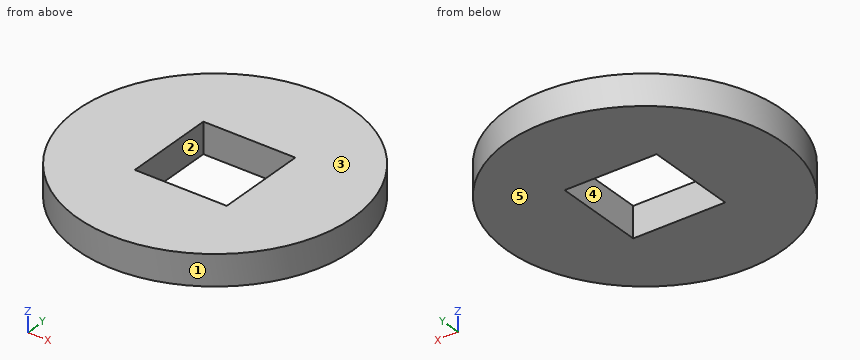
from build123d import *

# Parameters (mm, degrees)
SKETCH_1_R      = 4.5
SKETCH_1_W      = 3
SKETCH_1_H      = 3
EXTRUDE_1_DEPTH = 1


with BuildPart() as part:
    # 草图1 → 凸台-拉伸1 (new body)
    with BuildSketch(Plane.XY):
        Circle(SKETCH_1_R)
        Rectangle(SKETCH_1_W, SKETCH_1_H, mode=Mode.SUBTRACT)
    extrude(amount=EXTRUDE_1_DEPTH)


solid = part.part
Build history of the part. All positions in model axes, mm. Face numbers are marked on the shaded views. A direction names the side the tool comes from. Give positions to 0.01 mm unless a question says otherwise; leave off trailing zeros. Order: outer loops, then holes, each group sorted by start corner. A loop starts at its lowest first (then second) coordinate and runs counter-clockwise, first axis right, second up. Notation, with made-up numbers: M -18.5,20.25 L 7.5,20.25 A18 cw 7.5,42.25 Z; hole C -28,49.25 d1. An arc over 180 degrees is marked long. Put each result on its own line as item: value.
Item 1: Slice it at C-C, the plane z = 0.7. Write the cut outline in (x, y), plus the area to 3 significant figures.
From the geometry:
outline: C 0,0 d9; hole M -1.5,-1.5 L 1.5,-1.5 L 1.5,1.5 L -1.5,1.5 Z
area: 54.6 mm2
Item 2: Two-plate mould, pull along Y, no slides. Class the marked faces 1, 2 and 3: +Y half, -Y half, draft (parallel to the pull), parting line (faces both ways), or undercut.
From the geometry:
face 1: parting line
face 2: undercut
face 3: draft
Item 3: Flat gauge pin, fed straight in: pin 1 Ø5 at (x, y) = (-2.5, 2.5) entering from -Z. Where does the tip first touch, or does it go through?
From the geometry:
pin 1: stops at z = 0
Item 4: Probe line 1 (Y direction, x = -1, z = 0.6); line 2 (Y direction, x = 0, z = 0.8); line 3 (X direction, y = 0.25, z = 0.6). List the from-to ranges inside material, lowest first. Write a range as [from, to].
From the geometry:
line 1: y = [-4.39, -1.5], [1.5, 4.39]
line 2: y = [-4.5, -1.5], [1.5, 4.5]
line 3: x = [-4.49, -1.5], [1.5, 4.49]
Item 5: 3-axis set-ups, long thin cutter, end or side, ignore diameter. For the marked faces 4 and 5: which of +Z, -Z, +X, -X, +Y, -Y reach the whole face in a straight line?
From the geometry:
face 4: +Z, -Z
face 5: -Z, +X, -X, +Y, -Y
Item 6: Slice it at A-A, the plane y = 0. Write the cut outline in (x, z), plus the area to 3 significant figures.
From the geometry:
outline: M -4.5,0 L -1.5,0 L -1.5,1 L -4.5,1 Z; M 1.5,0 L 4.5,0 L 4.5,1 L 1.5,1 Z
area: 6.00 mm2
Item 7: Slice it at D-D, the plane y = -2.5. Write the cut outline in (x, z), plus the area to 3 significant figures.
From the geometry:
outline: M -3.74,0 L 3.74,0 L 3.74,1 L -3.74,1 Z
area: 7.48 mm2
